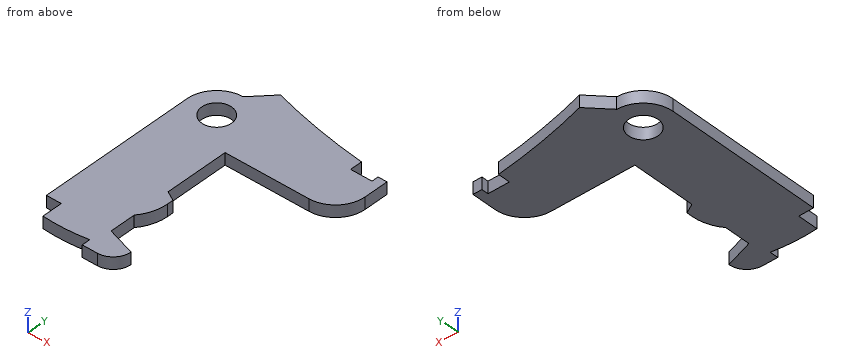
from build123d import *

# Parameters (mm, degrees)
SKETCH_1_R      = 2.5
EXTRUDE_1_DEPTH = 2


with BuildPart() as part:
    # 스케치1 → 보스-돌출1 (new body)
    with BuildSketch(Plane.XY):
        with BuildLine():
            Line((58.562856649, -69.110949309), (61.100431709, -69.110949309))
            ThreePointArc((61.100431709, -69.110949309), (63.221752053, -68.232269653), (64.100431709, -66.110949309))
            Line((64.100431709, -66.110949309), (59.376120264, -64.586771365))
            Line((59.376120264, -64.586771365), (59.376120264, -60.240028533))
            ThreePointArc((59.376120264, -60.240028533), (60.576391584, -58.13775418), (60.992924776, -55.753072063))
            Line((60.992924776, -55.753072063), (60.992924776, -54.755314285))
            Line((60.992924776, -54.755314285), (59.376120264, -53.867981647))
            Line((59.376120264, -53.867981647), (59.376120264, -43.149191929))
            Line((59.376120264, -43.149191929), (73.486715323, -43.149191929))
            ThreePointArc((73.486715323, -43.149191929), (77.022249229, -41.684725835), (78.486715323, -38.149191929))
            Line((78.486715323, -38.149191929), (78.486715323, -34.05327534))
            Line((78.486715323, -34.05327534), (76.986715323, -34.05327534))
            Line((76.986715323, -34.05327534), (76.986715323, -35.198463464))
            Line((76.986715323, -35.198463464), (73.386715323, -35.198463464))
            Line((73.386715323, -35.198463464), (73.386715323, -33.149191929))
            ThreePointArc((73.386715323, -33.149191929), (64.982885636, -31.8013595), (56.718627509, -29.765912799))
            Line((56.718627509, -29.765912799), (53.486715323, -33.149191929))
            ThreePointArc((53.486715323, -33.149191929), (49.951181417, -34.613658023), (48.486715323, -38.149191929))
            Line((48.486715323, -38.149191929), (48.486715323, -64.586869755))
            Line((48.486715323, -64.586869755), (50.986715323, -64.586869755))
            Line((50.986715323, -64.586869755), (50.986715323, -68.023666262))
            ThreePointArc((50.986715323, -68.023666262), (54.785213458, -68.09995351), (58.562856649, -67.695206989))
            Line((58.562856649, -67.695206989), (58.562856649, -69.110949309))
        make_face()
        with Locations((53.486715323, -38.149191929)):
            Circle(SKETCH_1_R, mode=Mode.SUBTRACT)
    extrude(amount=EXTRUDE_1_DEPTH)


solid = part.part
Design review of the part built by this model. Coordinates are the model's own, in mm. Round coordinates to 2 decimals unless told otherwise and drop trailing zeros. Write each loop counter-clockwise with the first axis right and the second up, starting at its lowest first coordinate (ties: lowest second). Pieces come first, ordered by that corner, then holes.
Item 1: Consider section B-B on y = -34.5. Give the boundary of the cut face in (x, z).
Item 2: Consider section C-C on x = 55.5. Give the boundary of the cut face in (y, z).
Item 3: Consider section D-D on y = -47. Give the boundary of the cut face in (x, z), and give its area (3 significant figures).
Item 4: Consider section A-A on z = 0.7. Give the boundary of the cut face in (x, y).
Item 5: Wall thickness on L1, parallel to X at y = -64, z = 0.35; L2, parallel to Y at x = 59.75, z = 1.45; L3, parallel to Y at x = 55.25, z = 1.4: over which ranges is each line inside the solid? List them lowest first.
Item 6: For pin 1 Ø0.6 at (y, z) = (-66, 1) entering from -X; pin 2 Ø0.5 at (y, z) = (-55.5, 1) entering from +X; pin 3 Ø12 at (x, y) = (72.5, -59) entering from -Z; pin 4 Ø0.6 at (y, z) = (-46, 1.5) entering from +X, all flat-tipped, find the tip position at first contact; note any pin that passes through.
Check values:
1. outline: (50.07, 0) - (73.39, 0) - (73.39, 2) - (50.07, 2) - close; (76.99, 0) - (78.49, 0) - (78.49, 2) - (76.99, 2) - close
2. outline: (-68.06, 0) - (-39.63, 0) - (-39.63, 2) - (-68.06, 2) - close; (-36.67, 0) - (-31.04, 0) - (-31.04, 2) - (-36.67, 2) - close
3. outline: (48.49, 0) - (59.38, 0) - (59.38, 2) - (48.49, 2) - close
3. area: 21.8 mm2
4. outline: (48.49, -64.59) - (50.99, -64.59) - (50.99, -68.02) arc R29.98 ccw to (58.56, -67.7) - (58.56, -69.11) - (61.1, -69.11) arc R3 ccw to (64.1, -66.11) - (59.38, -64.59) - (59.38, -60.24) arc R7.03 ccw to (60.99, -55.75) - (60.99, -54.76) - (59.38, -53.87) - (59.38, -43.15) - (73.49, -43.15) arc R5 ccw to (78.49, -38.15) - (78.49, -34.05) - (76.99, -34.05) - (76.99, -35.2) - (73.39, -35.2) - (73.39, -33.15) arc R103.25 cw to (56.72, -29.77) - (53.49, -33.15) arc R5 ccw to (48.49, -38.15) - close; hole circle Ø5 at (53.49, -38.15)
5. L1: x = 48.49 to 59.38
5. L2: y = -69.11 to -64.71, -59.75 to -54.07, -43.15 to -30.6
5. L3: y = -68.08 to -39.92, -36.38 to -31.3
6. pin 1: stops at x = 50.99
6. pin 2: stops at x = 60.99
6. pin 3: passes through
6. pin 4: stops at x = 59.38
